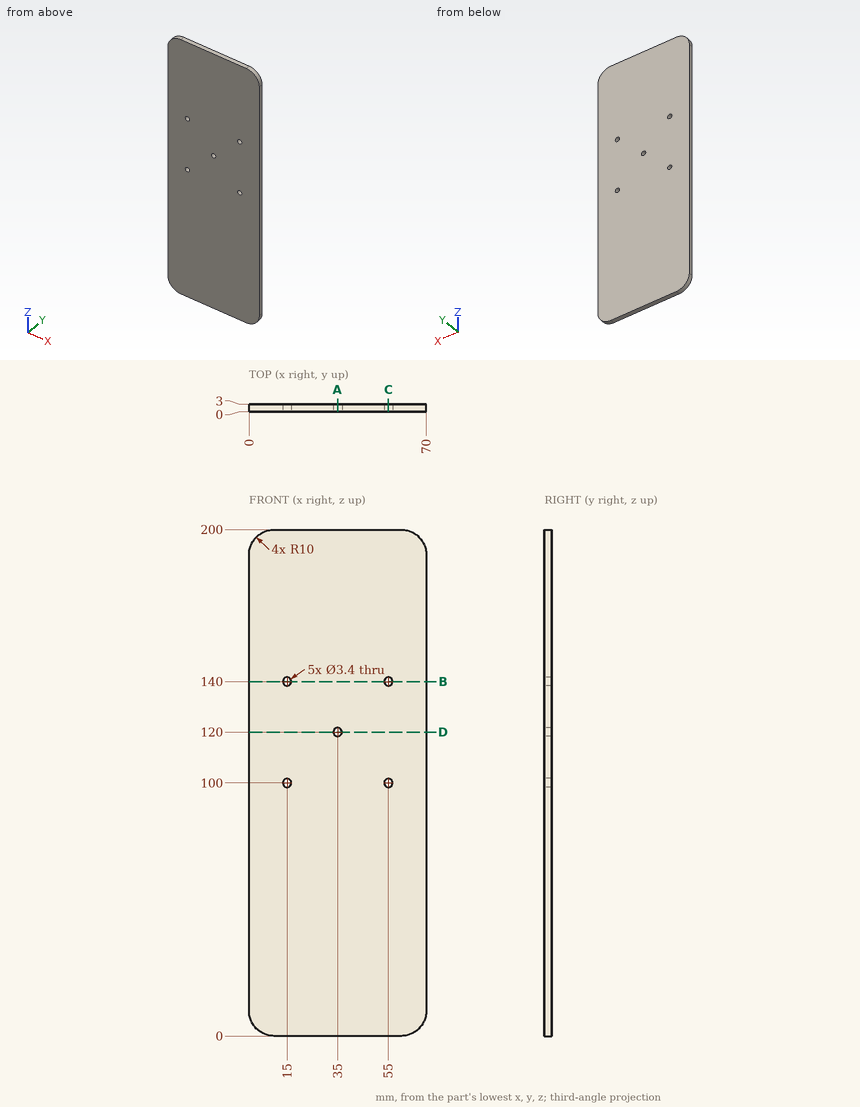
The figure shows three views and two pictorial views of one solid part (mm, origin at its lowest corner). Answer the questions. Coordinates: 2 decimals unless noted, no trailing zeros. Write each loop counter-clockwise with the first axis right and the second up, starting at its lowest first coordinate (ties: lowest second). Pieces come first, ordered by that corner, then holes. Notation, with made-up numbers: (-29.5, 85) -> (-5.5, 85) arc R24 ccw to (-5.5, 119) -> close; hole circle Ø10 at (-18.5, 58.5). An arc over 180 degrees is marked (long way). Return JSON: item names as keys, results as strings.
(1) Consider line 1 along X through (y, z) = (1.75, 100); line 2 along Z through (x, y) = (55, 2.2); line 3 along X through (y, z) = (1.4, 120). Determine where each line is inside the solid, lowest interval first. Write a range as from..to.
Answers below:
{"line 1": "0..13.3, 16.7..53.3, 56.7..70", "line 2": "0..98.3, 101.7..138.3, 141.7..200", "line 3": "0..33.3, 36.7..70"}
(2) The part is cut by section D-D on z = 120. Give the vertices of the cut face in (x, y), then the cut area to 3 significant figures.
Answers below:
{"outline": "(0, 0) -> (33.3, 0) -> (33.3, 3) -> (0, 3) -> close; (36.7, 0) -> (70, 0) -> (70, 3) -> (36.7, 3) -> close", "area": "200 mm^2"}
(3) The part is cut by section A-A on x = 35. Give the vertices of the cut face in (y, z), then the cut area to 3 significant figures.
Answers below:
{"outline": "(0, 0) -> (3, 0) -> (3, 118.3) -> (0, 118.3) -> close; (0, 121.7) -> (3, 121.7) -> (3, 200) -> (0, 200) -> close", "area": "590 mm^2"}
(4) The part is cut by section C-C on x = 55. Give the vertices of the cut face in (y, z), then the cut area to 3 significant figures.
Answers below:
{"outline": "(0, 0) -> (3, 0) -> (3, 98.3) -> (0, 98.3) -> close; (0, 101.7) -> (3, 101.7) -> (3, 138.3) -> (0, 138.3) -> close; (0, 141.7) -> (3, 141.7) -> (3, 200) -> (0, 200) -> close", "area": "580 mm^2"}
(5) The part is cut by section B-B on z = 140. Give the vertices of the cut face in (x, y), then the cut area to 3 significant figures.
Answers below:
{"outline": "(0, 0) -> (13.3, 0) -> (13.3, 3) -> (0, 3) -> close; (16.7, 0) -> (53.3, 0) -> (53.3, 3) -> (16.7, 3) -> close; (56.7, 0) -> (70, 0) -> (70, 3) -> (56.7, 3) -> close", "area": "190 mm^2"}
